from build123d import *

# Parameters (mm, degrees)
SKETCH1_R               = 4.15
SKETCH1_R_2             = 12.75
BOSS_EXTRUDE1_DEPTH     = 20
SKETCH2_R               = 16
SKETCH2_R_2             = 3.75
SKETCH2_R_3             = 1.5
BOSS_EXTRUDE2_DEPTH     = 2
SKETCH3_W               = 5.093214229
SKETCH3_H               = 2.005927174
CUT_EXTRUDE1_DEPTH      = 23
SKETCH5_R               = 1
CUT_EXTRUDE2_DEPTH      = 18.334595307
CUT_EXTRUDE2_DEPTH_BACK = 15.665404693


with BuildPart() as part:
    # Sketch1 → Boss-Extrude1 (new body)
    with BuildSketch(Plane.XY):
        with BuildLine():
            Line((-160.190785915, 7.025436305), (-21.138691228, 7.025436305))
            ThreePointArc((-21.138691228, 7.025436305), (-8.417687759, 10.994498434), (-21.063816819, 15.196022353))
            Line((-21.063816819, 15.196022353), (-160.043113059, 15.196022353))
            ThreePointArc((-160.043113059, 15.196022353), (-191.581294649, 11.679406985), (-160.190785915, 7.025436305))
        make_face()
        with Locations((-15.417393858, 11.05864302)):
            Circle(SKETCH1_R, mode=Mode.SUBTRACT)
        with Locations((-175.583907283, 11.39027474)):
            Circle(SKETCH1_R_2, mode=Mode.SUBTRACT)
    extrude(amount=BOSS_EXTRUDE1_DEPTH)

    # Sketch2 → Boss-Extrude2 (add)
    with BuildSketch(Plane(origin=(0, 0, 0), x_dir=(-1, 0, 0), z_dir=(0, 0, -1))):
        with Locations((175.583907283, 11.39027474)):
            Circle(SKETCH2_R)
        with Locations((175.583907283, 11.39027474)):
            Circle(SKETCH2_R_2, mode=Mode.SUBTRACT)
        with Locations((184.083907283, 11.39027474)):
            Circle(SKETCH2_R_3, mode=Mode.SUBTRACT)
        with Locations((167.083907283, 11.39027474)):
            Circle(SKETCH2_R_3, mode=Mode.SUBTRACT)
    extrude(amount=BOSS_EXTRUDE2_DEPTH)

    # Sketch3 → Cut-Extrude1 (cut, through all)
    with BuildSketch(Plane.XY.offset(20)):
        with Locations((-9.977016533, 11.05864302)):
            Rectangle(SKETCH3_W, SKETCH3_H)
    extrude(amount=-CUT_EXTRUDE1_DEPTH, mode=Mode.SUBTRACT)

    # Sketch5 → Cut-Extrude2 (cut, two sides)
    with BuildSketch(Plane(origin=(0, 10.055679433, 0), x_dir=(1, 0, 0), z_dir=(0, 1, 0))) as cut_extrude2_sk:
        with Locations((-9.962338035, -10.18638419)):
            Circle(SKETCH5_R)
    extrude(amount=CUT_EXTRUDE2_DEPTH, mode=Mode.SUBTRACT)
    extrude(cut_extrude2_sk.sketch, amount=-CUT_EXTRUDE2_DEPTH_BACK, mode=Mode.SUBTRACT)


solid = part.part
Geometry check sheet. Reference: the model listing, model coordinates, mm. A direction names the side the tool comes from. Give positions to 0.01 mm unless a question says otherwise; leave off trailing zeros. Loops run counter-clockwise (first coordinate to the right, second up) from the corner with the lowest first, then second, coordinate; pieces in that order, holes last. Notation, with made-up numbers: M 64,78.5 L 83,78.5 A28 ccw 83,110.5 Z; hole C 68,50.25 d2. An arc over 180 degrees is marked long. Answer as a JSON object with one key per item and string values. Group by question number.
Item 1: Mould release check, pull along Y, two halves, no side actions. Record for faces 6 (the cylindrical face through (-19.564, 11.227, 9.86)), 7 (the cylindrical face through (-163.423, 15.22, 9.86)), 8 (the cylindrical face through (-13.61, 17.82, 9.86)), 9 (the flat face through (-179, 8, -2)): pulls with the +Y half, pulls with the -Y half, needs draft (parallel to the pull), parting line crosses it, or undercut.
Item 2: Sectioned sample at A-A on z = 2. Record the boundary of the cut face in (x, y), plus the area to 3 significant figures.
Item 3: Sectioned sample at D-D on y = 0.5. Record the boundary of the cut face in (x, z).
Item 4: Gauge pin test, flat ends, axial feed: pin 1 (2 mm diameter, centred on y = 14, z = 0.5, fed in from -X); pin 2 (8 mm diameter, centred on y = 2, z = 0.5, fed in from -X); pin 3 (7 mm diameter, centred on x = -54.5, y = 12, fed in from -Z); pin 4 (13.5 mm diameter, centred on x = -15.42, y = 11.06, fed in from +Z). Record the tip position at first contact, or that the pin passes through.
Item 5: Material ranges on L1, parallel to X at y = 5.5, z = 10.75; L2, parallel to X at y = 13.5, z = 12; L3, parallel to X at y = 11.5, z = 10.25, recorded low to high.
Item 6: Sectioned sample at C-C on x = -147.5. Record the boundary of the cut face in (y, z).
Item 7: Access from +Z, -Z, +X, -X, +Y, -Y to the whole of each face (thin tool, end or side, straight path). Record for faces 1 (the flat face through (-85, 11, 0)), 2 (the flat face through (-92, 7.025, 10)), 3 (the flat face through (-90, 15.196, 10)), 4 (the flat face through (-11.2, 10.056, 10.1)), 5 (the flat face through (-172.6, 8.7, 0)).
Item 8: Sectioned sample at B-B on y = 21.5. Record the boundary of the cut face in (x, z) (3 decimals).
Findings below:
{
 "1": {"face 6": "undercut", "face 7": "undercut", "face 8": "pulls with the +Y half", "face 9": "needs draft"},
 "2": {"outline": "M -160.19,7.03 L -21.14,7.03 A7 ccw -8.49,10.06 L -11.39,10.06 A4.15 cw long -11.39,12.06 L -8.49,12.06 A7 ccw -21.06,15.2 L -160.04,15.2 A16 ccw long Z; hole C -175.58,11.39 d25.5", "area": "1,510 mm2"},
 "3": {"outline": "M -187.31,-2 L -163.86,-2 L -163.86,20 L -168.95,20 L -168.95,0 L -182.21,0 L -182.21,20 L -187.31,20 Z"},
 "4": {"pin 1": "x = -191.5", "pin 2": "x = -190.65", "pin 3": "z = 0", "pin 4": "z = 20"},
 "5": {"L1": "-190.46 to -186.89, -164.28 to -160.71, -19.67 to -11.16", "L2": "-191.44 to -188.16, -163.01 to -18.77, -12.06 to -8.86", "L3": "-191.58 to -188.33, -162.83 to -19.54"},
 "6": {"outline": "M 7.03,0 L 15.2,0 L 15.2,20 L 7.03,20 Z"},
 "7": {"face 1": "-Z, +X, +Y, -Y", "face 2": "+Z, -Z, -Y", "face 3": "+Z, -Z, +Y", "face 4": "+Z, -Z, +X", "face 5": "+Z"},
 "8": {"outline": "M -187.985,-2 L -163.183,-2 L -163.183,20 L -167.815,20 L -167.815,0 L -183.353,0 L -183.353,20 L -187.985,20 Z"}
}
